Build history of the part. All positions in model axes, mm. Coordinates: 2 decimals unless noted, no trailing zeros. Loops run counter-clockwise (first coordinate to the right, second up) from the corner with the lowest first, then second, coordinate; pieces in that order, holes last. Notation, with made-up numbers: (3, 63.5) -> (34, 63.5) arc R28 cw to (34, 90.5) -> close; hole circle Ø4 at (37.25, 36). An arc over 180 degrees is marked (long way). One line per item, written item: value. Start each with the question number.
```python
from build123d import *

# Parameters (mm, degrees)
SKETCH2_R           = 2.4892
BOSS_EXTRUDE1_DEPTH = 3.175
LPATTERN1_OUTLINE_R = 2.4892
LPATTERN1_DEPTH     = 3.175
CUT_EXTRUDE1_DEPTH  = 124.335571207
FILLET2_R           = 6.35


# Read off the part's stored shape, not the designer's step: LPattern1
with BuildPart() as part:
    # Sketch2 → Boss-Extrude1 (new body)
    with BuildSketch(Plane(origin=(0, 0, 0), x_dir=(1, 0, 0), z_dir=(0, 1, 0))):
        Polygon((0, 0), (0, 101.6), (-25.4, 101.6), (-69.85, 25.4), (-69.85, 0), align=None)
        with Locations(Location((-12.7, 12.7, 0), (0, 0, 270))):
            Circle(SKETCH2_R, mode=Mode.SUBTRACT)
    extrude(amount=BOSS_EXTRUDE1_DEPTH)

    # LPattern1 outline → LPattern1 (cut)
    with BuildSketch(Plane(origin=(0, 0, 0), x_dir=(1, 0, 0), z_dir=(0, 1, 0))):
        with Locations((-63.5, 12.7)):
            Circle(LPATTERN1_OUTLINE_R)
        with Locations((-50.8, 12.7)):
            Circle(LPATTERN1_OUTLINE_R)
        with Locations((-38.1, 12.7)):
            Circle(LPATTERN1_OUTLINE_R)
        with Locations((-25.4, 12.7)):
            Circle(LPATTERN1_OUTLINE_R)
        with Locations((-12.7, 88.9)):
            Circle(LPATTERN1_OUTLINE_R)
        with Locations((-12.7, 76.2)):
            Circle(LPATTERN1_OUTLINE_R)
        with Locations((-12.7, 63.5)):
            Circle(LPATTERN1_OUTLINE_R)
        with Locations((-12.7, 50.8)):
            Circle(LPATTERN1_OUTLINE_R)
        with Locations((-12.7, 38.1)):
            Circle(LPATTERN1_OUTLINE_R)
        with Locations((-12.7, 25.4)):
            Circle(LPATTERN1_OUTLINE_R)
    extrude(amount=LPATTERN1_DEPTH, mode=Mode.SUBTRACT)

    # Sketch3 → Cut-Extrude1 (cut, through all)
    with BuildSketch(Plane(origin=(0, 3.175, 0), x_dir=(1, 0, 0), z_dir=(0, 1, 0))):
        Polygon((-7.62, 31.75), (0, 39.37), (0, 31.75), (0, 0), (-7.62, 0), align=None)
    extrude(amount=-CUT_EXTRUDE1_DEPTH, mode=Mode.SUBTRACT)

    # Fillet2
    fillet2_edges = [part.edges().sort_by_distance(p)[0] for p in [
        (-7.62, 1.5875, 0),
        (-7.62, 1.5875, -31.75),
        (0, 1.5875, -39.37),
        (-69.85, 1.5875, 0),
        (-69.85, 1.5875, -25.4),
        (-25.4, 1.5875, -101.6),
        (0, 1.5875, -101.6),
    ]]
    fillet(fillet2_edges, radius=FILLET2_R)


solid = part.part
```
Item 1: Two-plate mould, pull along Z, no slides. Class faces 1 (the face through (-11.551, 1.565, -35.892)), 2 (the face through (-69.636, 1.61, -25.318)), 3 (the face through (0, 2, -68)): +Z half, -Z half, draft (parallel to the pull), parting line (faces both ways), or undercut.
Item 2: Band-saw the part on A-A, the plane z = -25.4. List the corners of the cut face in (x, y) (3 decimals).
Item 3: Band-saw the part on D-D, the plane z = -11.5. List the corners of the cut face in (x, y) (3 decimals).
Item 4: Probe probe 1 along X at (y, z) = (0.7, -12.7); probe 2 along X at (y, z) = (1, -13.5); probe 3 along X at (y, z) = (0.35, -17). List the from-to ranges inside material, lowest first.
Item 5: Drop flat-ended pins along their axis: pin 1 Ø1 at (y, z) = (2, -16.5) entering from +X; pin 2 Ø1 at (x, y) = (-12, 2.5) entering from +Z. Give the stop position or say it passes through.
Item 6: Band-saw the part on B-B, the plane x = -24. List the corners of the cut face in (y, z) (3 decimals).
Item 7: Band-saw the part on C-C, the plane y = 0.7. Count the separate pieces of the cut face and the enclosed holes in it, and give its area (3 significant figures).
Worked out:
1. face 1: undercut
1. face 2: -Z half
1. face 3: draft
2. outline: (-69.614, 0) -> (-15.189, 0) -> (-15.189, 3.175) -> (-69.614, 3.175) -> close; (-10.211, 0) -> (-7.62, 0) -> (-7.62, 3.175) -> (-10.211, 3.175) -> close
3. outline: (-69.85, 0) -> (-65.681, 0) -> (-65.681, 3.175) -> (-69.85, 3.175) -> close; (-61.319, 0) -> (-52.981, 0) -> (-52.981, 3.175) -> (-61.319, 3.175) -> close; (-48.619, 0) -> (-40.281, 0) -> (-40.281, 3.175) -> (-48.619, 3.175) -> close; (-35.919, 0) -> (-27.581, 0) -> (-27.581, 3.175) -> (-35.919, 3.175) -> close; (-23.219, 0) -> (-14.881, 0) -> (-14.881, 3.175) -> (-23.219, 3.175) -> close; (-10.519, 0) -> (-7.62, 0) -> (-7.62, 3.175) -> (-10.519, 3.175) -> close
4. probe 1: x = -69.85 to -65.99, -61.01 to -53.29, -48.31 to -40.59, -35.61 to -27.89, -22.91 to -15.19, -10.21 to -7.62
4. probe 2: x = -69.85 to -65.86, -61.14 to -53.16, -48.44 to -40.46, -35.74 to -27.76, -23.04 to -15.06, -10.34 to -7.62
4. probe 3: x = -69.85 to -7.62
5. pin 1: stops at x = -7.62
5. pin 2: stops at z = -0.17
6. outline: (0, -101.189) -> (3.175, -101.189) -> (3.175, -14.758) -> (0, -14.758) -> close; (0, -10.642) -> (3.175, -10.642) -> (3.175, 0) -> (0, 0) -> close
7. separate pieces: 1
7. enclosed holes: 11
7. area: 4,890 mm²
